from build123d import *

# Parameters (mm, degrees)
SKETCH_R        = 1.55
PAD_DEPTH       = 6.3
SKETCH002_W     = 5.6
SKETCH002_H     = 5.6
POCKET_DEPTH    = 2
PAD001_DEPTH    = 7.7
SKETCH003_R     = 1.65
POCKET001_DEPTH = 4.901
SKETCH004_W     = 5.6
SKETCH004_H     = 5.6
POCKET002_DEPTH = 2
SKETCH005_W     = 8
SKETCH005_H     = 7
PAD002_DEPTH    = 11.9
SKETCH006_R     = 1.6
PAD003_DEPTH    = 7.5
PAD004_DEPTH    = 11.9
FILLET_R        = 5
CHAMFER_SIZE    = 5.5


with BuildPart() as part:
    # Sketch → Pad (new body)
    with BuildSketch(Plane.YZ):
        Polygon((-4.9, -4.5), (0, -4.5), (0, -19), (-15, -19), (-15, -11), (-4.9, -11), align=None)
        with Locations((-11, -15)):
            Circle(SKETCH_R, mode=Mode.SUBTRACT)
        with Locations((-4, -15)):
            Circle(SKETCH_R, mode=Mode.SUBTRACT)
    extrude(amount=PAD_DEPTH)

    # Sketch002 (on Face9 of Pad) → Pocket (cut)
    with BuildSketch(Plane(origin=(0, 0, 0), x_dir=(0, 1, 0), z_dir=(-1, 0, 0))):
        with Locations((-11, 15)):
            Rectangle(SKETCH002_W, SKETCH002_H)
        with Locations((-4, 15)):
            Rectangle(SKETCH002_W, SKETCH002_H)
    extrude(amount=-POCKET_DEPTH, mode=Mode.SUBTRACT)

    # Sketch001 (on Face1 of Pad) → Pad001 (join)
    with BuildSketch(Plane(origin=(0, 0, -4.5), x_dir=(0, -1, 0), z_dir=(0, 0, 1))):
        Polygon((0, 0), (0, -16), (8, -16), (8, -9), (4.9, -9), (4.9, -2.7), (8, -2.7), (8, 0), align=None)
    extrude(amount=-PAD001_DEPTH)

    # Sketch003 (on Face1 of Pad001) → Pocket001 (cut, through all)
    with BuildSketch(Plane(origin=(0, -4.9, 0), x_dir=(0, 0, -1), z_dir=(0, -1, 0))):
        with Locations((8.15, -5.85)):
            Circle(SKETCH003_R)
        with Locations((8.15, 3.15)):
            Circle(SKETCH003_R)
    extrude(amount=-POCKET001_DEPTH, mode=Mode.SUBTRACT)

    # Sketch004 (on Face10 of Pocket001) → Pocket002 (cut)
    with BuildSketch(Plane.ZX):
        with Locations((-8.15, 3.15)):
            Rectangle(SKETCH004_W, SKETCH004_H)
        with Locations((-8.15, -5.85)):
            Rectangle(SKETCH004_W, SKETCH004_H)
    extrude(amount=-POCKET002_DEPTH, mode=Mode.SUBTRACT)

    # Sketch005 (on Face5 of Pocket002) → Pad002 (join)
    with BuildSketch(Plane(origin=(0, 0, -4.5), x_dir=(0, -1, 0), z_dir=(0, 0, 1))):
        with Locations((4, -12.5)):
            Rectangle(SKETCH005_W, SKETCH005_H)
    extrude(amount=PAD002_DEPTH)

    # Sketch006 (on Face36 of Pad002) → Pad003 (join)
    with BuildSketch(Plane(origin=(0, -8, 0), x_dir=(0, 0, -1), z_dir=(0, -1, 0))):
        with Locations((-2.05, -12.7)):
            Circle(SKETCH006_R)
        with Locations((2.05, -12.7)):
            Circle(SKETCH006_R)
    extrude(amount=PAD003_DEPTH)

    # Sketch007 → Pad004 (join)
    with BuildSketch(Plane(origin=(0, 0, -4.5), x_dir=(0, -1, 0), z_dir=(0, 0, 1))):
        with BuildLine():
            Line((8, -2.5), (1.15, -2.5))
            ThreePointArc((1.15, -0.2), (0, -1.35), (1.15, -2.5))
            Line((1.15, -0.2), (8, -0.2))
            Line((8, -0.2), (8, -2.5))
        make_face()
    extrude(amount=PAD004_DEPTH)

    # Fillet
    fillet_edges = [part.edges().sort_by_distance(p)[0] for p in [
        (-16, -4, 7.4),
    ]]
    fillet(fillet_edges, radius=FILLET_R)

    # Chamfer
    chamfer_edges = [part.edges().sort_by_distance(p)[0] for p in [
        (-16, -4, -12.2),
    ]]
    chamfer(chamfer_edges, length=CHAMFER_SIZE)


solid = part.part
Geometry: final body of the model. Coordinates: model frame, mm. A direction names the side the tool comes from. Round coordinates to 2 decimals unless told otherwise and drop trailing zeros. Order: outer loops, then holes, each group sorted by start corner. A loop starts at its lowest first (then second) coordinate and runs counter-clockwise, first axis right, second up. Notation, with made-up numbers: (-0.5, -0.75) -> (14.5, -0.75) arc R24 ccw to (14.5, 13.25) -> close; hole circle Ø11 at (37.5, 61.5). An arc over 180 degrees is marked (long way). Put each result on its own line as item: value. Start each with the question number.
Q1. Section A-A on x = 3.15. Return the cut outline in (y, z), and give its area (3 significant figures).
Q2. Reachability of faces 4 (the flat face through (2, -12.3, -16.3)), 5 (the flat face through (3, -1, -5.35)), 6 (the flat face through (-0.2, -5, 1)), 7 (the flat face through (-2.5, -5, 1)) from +Z, -Z, +X, -X, +Y, -Y: full face, straight path, thin tool, end or side. Return the list, or none.
Q3. First-contact query: pin 1 (6 mm diameter, centred on x = -10.5, z = 1.5, fed in from -Y); pin 2 (0.6 mm diameter, centred on x = 0.5, z = -14.5, fed in from -Y); pin 3 (4 mm diameter, centred on y = -6.5, z = -16, fed in from -X); pin 4 (5 mm diameter, centred on y = -11, z = -15, fed in from -X). Flat tips, straight axial feed; report the tip coordinate or a pass-through.
Q4. Line query: probe 1 along Y at (x, z) = (3.4, -15); probe 2 along Z at (x, y) = (5.4, -4); probe 3 along X at (y, z) = (-5.75, -5.5). Output: solid intervals per line, ascending.
Q5. Section C-C on z = -8.15. Return the cut outline in (x, y).
Q6. Section D-D on z = -5. Return the cut outline in (x, y).
Q7. Pull-direction query (Z, two-part tool) for faces 1 (the flat face through (-10, 0, -6)), 2 (the flat face through (-5, -3, -4.5)), 3 (the flat face through (-8.65, -1, -8)); classes: +Z half, -Z half, draft (parallel to the pull), parting line (faces both ways), or undercut.
Q8. Section B-B on y = -11. Return the cut outline in (x, z).
Ans:
1. outline: (-15, -19) -> (0, -19) -> (0, -10.95) -> (-2, -10.95) -> (-2, -9.8) -> (-4.9, -9.8) -> (-4.9, -11) -> (-15, -11) -> close; (-4.9, -6.5) -> (-2, -6.5) -> (-2, -5.35) -> (0, -5.35) -> (0, -4.5) -> (-4.9, -4.5) -> close; hole circle Ø3.1 at (-11, -15); hole circle Ø3.1 at (-4, -15)
1. area: 116 mm2
2. face 4: -X
2. face 5: +Y
2. face 6: +Z, +X, +Y, -Y
2. face 7: +Z, +Y, -Y
3. pin 1: stops at y = -15.5
3. pin 2: stops at y = -15
3. pin 3: stops at x = 0
3. pin 4: stops at x = 2
4. probe 1: y = -15 to -12.55, -9.45 to -5.55, -2.45 to 0
4. probe 2: z = -19 to -16.55, -13.45 to -4.5
4. probe 3: x = -16 to -9, -2.7 to 0
5. outline: (-14.55, -8) -> (-9, -8) -> (-9, -4.9) -> (-7.5, -4.9) -> (-7.5, -2) -> (-8.65, -2) -> (-8.65, 0) -> (-14.55, 0) -> close; (-4.2, -4.9) -> (-2.7, -4.9) -> (-2.7, -8) -> (0, -8) -> (0, -4.9) -> (1.5, -4.9) -> (1.5, -2) -> (0.35, -2) -> (0.35, 0) -> (-3.05, 0) -> (-3.05, -2) -> (-4.2, -2) -> close; (4.8, -4.9) -> (6.3, -4.9) -> (6.3, 0) -> (5.95, 0) -> (5.95, -2) -> (4.8, -2) -> close
6. outline: (-16, -8) -> (-9, -8) -> (-9, -4.9) -> (-2.7, -4.9) -> (-2.7, -8) -> (0, -8) -> (0, -4.9) -> (6.3, -4.9) -> (6.3, 0) -> (-16, 0) -> close
7. face 1: draft
7. face 2: +Z half
7. face 3: undercut
8. outline: circle Ø3.2 at (-12.7, -2.05); circle Ø3.2 at (-12.7, 2.05); (0, -19) -> (6.3, -19) -> (6.3, -16.55) -> (2, -16.55) -> (2, -17.8) -> (0, -17.8) -> close; (0, -12.2) -> (2, -12.2) -> (2, -13.45) -> (6.3, -13.45) -> (6.3, -11) -> (0, -11) -> close
